Design review of the part built by this model. Coordinates are the model's own, in mm. A direction names the side the tool comes from. Coordinates: 2 decimals unless noted, no trailing zeros. Loops run counter-clockwise (first coordinate to the right, second up) from the corner with the lowest first, then second, coordinate; pieces in that order, holes last. Notation, with made-up numbers: (10, 26.5) -> (65, 26.5) arc R18 ccw to (65, 61.5) -> close; hole circle Ø8 at (42.5, -1). An arc over 180 degrees is marked (long way). Use one line per item in the form item = value. Start each with the question number.
1. The part is to be moulded in two halves that separate along Z. For faces 1 (the face through (-7, 18, -120.65)), 2 (the face through (-7, 16, 0)), 3 (the face through (-14.351, 6, -63)), say which applies: released by +Z, released by -Z, zero draft, split by the parting line, or undercut.
2. Consider section D-D (x = -1.25). State how many separate pieces and enclosed holes the cut face has, then the cut area to 3 significant figures.
3. Consider section A-A (z = -114.3). State the section outline as (x, y) points.
4. Consider section C-C (y = 27). State the section outline as (x, z) points, then the cut area to 3 significant figures.
5. Wall thickness on line 1 (Z direction, x = -8.75, y = 16.5); line 2 (Z direction, x = -6.5, y = 6); line 3 (Y direction, x = -0.5, z = -104.5): over which ranges is each line inside the solid? List them lowest first. Write a range as from..to.
6. Consider section B-B (y = 6.35). State the section outline as (x, z) points.
7. For pin 1 (5 mm diameter, centred on x = -13, z = -97.5, fed in from +Y); pin 2 (11 mm diameter, centred on y = 6.35, z = -12.7, fed in from +X); pin 3 (14 mm diameter, centred on y = 6, z = -41.5, fed in from -X), all flat-tipped, find the tip position at first contact; note any pin that passes through.
8. Machinability: for faces 4 (the face through (-6.8, 31.85, -3.13)), 5 (the face through (-10, 20, -6.35)), which of the approach directions +Z, -Z, +X, -X, +Y, -Y give a long, thin tool a straight path to every point of the face, cutting with its end or side? Answer none if there is none.
Autodesk Inventor part; units mm, degrees
ref_plane "Work Plane1" through (-14.351, 0, -63.5) normal (0, 0, 1) x (1, 0, 0)
ref_plane "YZ Plane" through (0, 0, 0) normal (1, 0, 0) x (0, 1, 0)
ref_plane "XZ Plane" through (0, 0, 0) normal (0, 1, 0) x (-1, 0, 0)
sketch "Sketch1" plane through (0, 0, 0) normal (0, 1, 0) x (-1, 0, 0)
  line L0 (0, 0) -> (14.351, 0)
  line L1 (14.351, 0) -> (14.351, -127)
  line L2 (14.351, -127) -> (0, -127)
  line L3 (0, -127) -> (0, 0)
  dimension "d0" = 127
  dimension "d1" = 14.351
extrude "Extrusion1" add sketch "Sketch1" along normal blind 12.7
sketch "Sketch2" plane through (0, 0, 0) normal (1, 0, 0) x (0, 0, -1)
  circle A0 centre (12.7, 6.35) radius 4.7625
  circle A1 centre (114.3, 6.35) radius 4.7625
  line L0 (0, 12.7) -> (127, 12.7)
  line L1 (127, 0) -> (127, 12.7)
  point P0 (0, 0)
  dimension "d4" = 9.525
  dimension "d5" = 9.525
  dimension "d6" = 101.6
  dimension "d7" = 127
  dimension "d8" = 12.7
  dimension "d9" = 12.7
  dimension "d10" = 6.35
  dimension "d11" = 6.35
extrude "Extrusion2" cut sketch "Sketch2" against normal through all
sketch "Sketch3" plane through (-14.351, 0, 0) normal (0, 0, 1) x (1, 0, 0)
  line L0 (0, 12.7) -> (14.351, 12.7)
  circle A0 centre (7.1755, 22.3312) radius 9.525
  circle A1 centre (7.1755, 29.9512) radius 0.5953
  circle A2 centre (-0.4445, 22.3312) radius 0.5953
  circle A3 centre (14.7955, 22.3312) radius 0.5953
  circle A4 centre (7.1755, 14.7112) radius 0.5953
  line L1 (14.351, 0) -> (14.351, 12.7)
  line L2 (0, 0) -> (0, 12.7)
  arc A5 (14.351, 12.7) -> (0, 12.7) centre (7.1755, 20.9342) ccw
  circle A6 centre (7.1755, 22.3312) radius 3.175
  dimension "d15" = 19.05
  dimension "d16" = 1.1906
  dimension "d17" = 1.1906
  dimension "d18" = 1.1906
  dimension "d19" = 1.1906
  dimension "d20" = 7.62
  dimension "d28" = 0
  dimension "d29" = 10.922
  dimension "d32" = 6.35
  dimension "d33" = 7.62
  dimension "d34" = 7.62
  dimension "d35" = 7.62
  dimension "d36" = 0
  dimension "d37" = 9.6312
  dimension "d38" = 0
  dimension "d39" = 0
  dimension "d40" = 0
ref_plane "Work Plane1" through (-14.351, 0, -63.5) normal (0, 0, 1) x (1, 0, 0)
extrude "Extrusion4" add sketch "Sketch3" against normal blind 6.35 contours A0 | A5 L0
mirror "Mirror1" about plane through (-14.351, 0, -63.5) normal (0, 0, 1) of "Extrusion4"
equation "\"d5\" = d4"
equation "\"d8\" = -0.5 * d6 + 0.5 * d7"
equation "\"d10\" = 0.5 * d9"
equation "\"d11\" = d10"
equation "\"d17\" = d16"
equation "\"d18\" = d17"
equation "\"d19\" = d17"
properties part number "axil mount"
Geometry check:
q1.face_1 = undercut
q1.face_2 = released by +Z
q1.face_3 = zero draft
q2.separate_pieces = 1
q2.enclosed_holes = 2
q2.area = 1,690 mm²
q3.outline = (-14.35, 0) -> (0, 0) -> (0, 1.59) -> (-14.35, 1.59) -> close; (-14.35, 11.11) -> (0, 11.11) -> (0, 12.7) -> (-14.35, 12.7) -> close
q4.outline = (-16.26, -127) -> (1.91, -127) -> (1.91, -120.65) -> (-16.26, -120.65) -> close; (-16.26, -6.35) -> (1.91, -6.35) -> (1.91, 0) -> (-16.26, 0) -> close
q4.area = 231 mm²
q5.line_1 = -127..-120.65, -6.35..0
q5.line_2 = -127..-119.05, -109.55..-17.45, -7.95..0
q5.line_3 = 0..12.7
q6.outline = (-14.35, -127) -> (0, -127) -> (0, -119.06) -> (-14.35, -119.06) -> close; (-14.35, -109.54) -> (0, -109.54) -> (0, -17.46) -> (-14.35, -17.46) -> close; (-14.35, -7.94) -> (0, -7.94) -> (0, 0) -> (-14.35, 0) -> close
q7.pin_1 = 12.7
q7.pin_2 = 0
q7.pin_3 = -14.35
q8.face_4 = +Z, -Z
q8.face_5 = +X, -X, +Y
